Could you check a few things on this drawing? It's one solid part, dimensions in mm from its lowest x, y, z. A direction names the side the tool comes from. Give positions to 0.01 mm unless a question says otherwise; leave off trailing zeros. Loops run counter-clockwise (first coordinate to the right, second up) from the corner with the lowest first, then second, coordinate; pieces in that order, holes last. Notation, with made-up numbers: (7, 34) - (37, 34) arc R13 ccw to (37, 50) - close; hole circle Ø6 at (89.25, 61.5). An arc over 180 degrees is marked (long way). Write item = value, one per line.
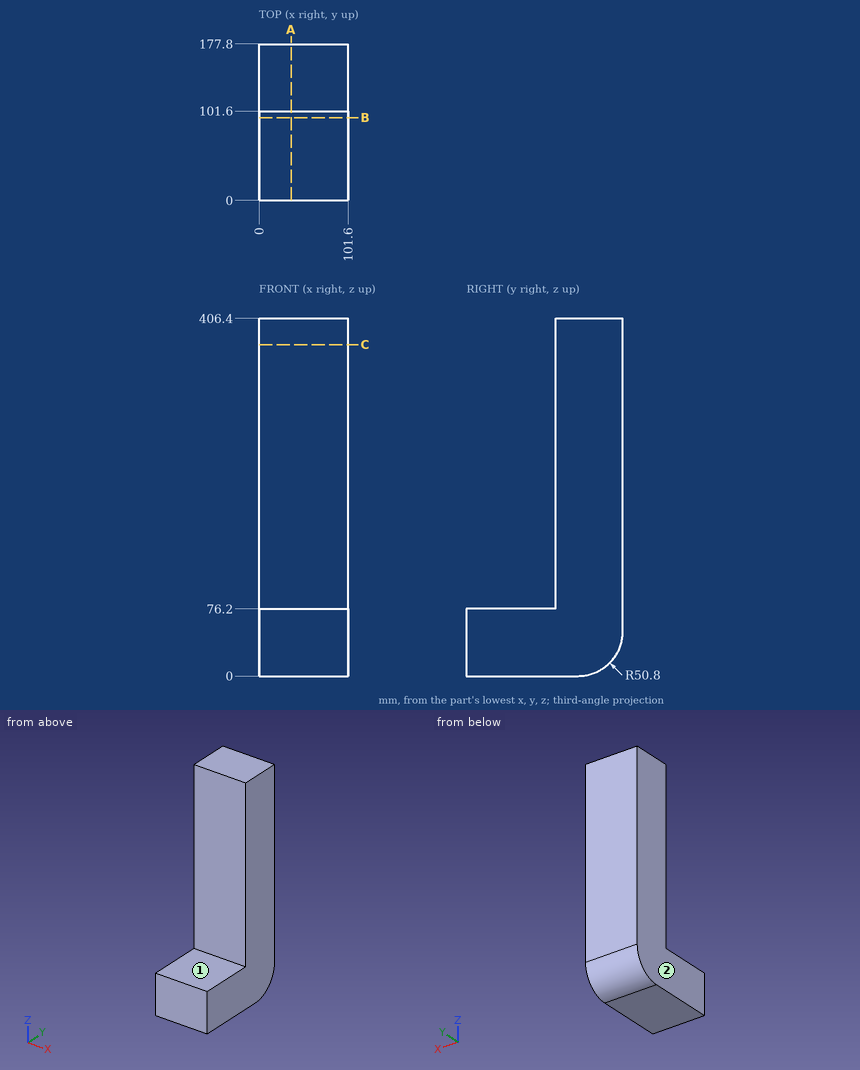
Q1. Imagine slicing it at B-B, the plane y = 94. Write out the boundary of the cut face in (x, z).
Output:
outline = (0, 0) - (101.6, 0) - (101.6, 76.2) - (0, 76.2) - close
Q2. For pin 1 (1 mm diameter, centred on x = 20, z = 267.5, fed in from -Y); pin 2 (3 mm diameter, centred on x = 51.5, y = 137.5, fed in from -Z), each with a flat end and sliding along its axis, tell me the tip position at first contact or that it passes through.
Output:
pin_1 = 101.6
pin_2 = 0.8
Q3. Imagine slicing it at A-A, the plane x = 36.5. Write out the boundary of the cut face in (y, z), then the cut area to 3 significant figures.
Output:
outline = (0, 0) - (127, 0) arc R50.8 ccw to (177.8, 50.8) - (177.8, 406.4) - (101.6, 406.4) - (101.6, 76.2) - (0, 76.2) - close
area = 38,200 mm2
Q4. I need wall thicknesses on L1, parallel to Z at x = 73.5, y = 99.5; L2, parallel to Y at x = 97.5, z = 152; L3, parallel to Z at x = 60, y = 143. Which ranges of each line are inside material? Lowest first, please.
Output:
L1 = 0 to 76.2
L2 = 101.6 to 177.8
L3 = 2.59 to 406.4
Q5. Which directions (+Z, -Z, +X, -X, +Y, -Y) give clear straight access to the entire face, cutting with the end or side of a thin tool? Please do the marked faces 1 and 2.
Output:
face_1 = +Z, +X, -X, -Y
face_2 = +Z, -Z, -X, +Y, -Y
Q6. Imagine slicing it at C-C, the plane z = 376.5. Write out the boundary of the cut face in (x, y), then the cut area to 3 significant figures.
Output:
outline = (0, 101.6) - (101.6, 101.6) - (101.6, 177.8) - (0, 177.8) - close
area = 7,740 mm2
